The model under review builds one solid part; all positions refer to its coordinate system, in mm. Round coordinates to 2 decimals unless told otherwise and drop trailing zeros.
```python
from build123d import *

# Parameters (mm, degrees)
SKETCH1_W           = 368.3
SKETCH1_H           = 292.1
SKETCH1_R           = 99.3775
SKETCH1_R_2         = 2.54
BOSS_EXTRUDE1_DEPTH = 6.35
SKETCH2_R           = 14.2875
SKETCH2_R_2         = 2.38125
CUT_EXTRUDE1_DEPTH  = 7.35
FILLET1_R           = 12.7


with BuildPart() as part:
    # Sketch1 → Boss-Extrude1 (new body)
    with BuildSketch(Plane.XY):
        with Locations((184.15, 146.05)):
            Rectangle(SKETCH1_W, SKETCH1_H)
        with Locations((179.07, 138.43)):
            Circle(SKETCH1_R, mode=Mode.SUBTRACT)
        with Locations((12.7, 279.4)):
            Circle(SKETCH1_R_2, mode=Mode.SUBTRACT)
        with Locations((25.4, 279.4)):
            Circle(SKETCH1_R_2, mode=Mode.SUBTRACT)
        with Locations((38.1, 279.4)):
            Circle(SKETCH1_R_2, mode=Mode.SUBTRACT)
        with Locations((50.8, 279.4)):
            Circle(SKETCH1_R_2, mode=Mode.SUBTRACT)
        with Locations((63.5, 279.4)):
            Circle(SKETCH1_R_2, mode=Mode.SUBTRACT)
        with Locations((76.2, 279.4)):
            Circle(SKETCH1_R_2, mode=Mode.SUBTRACT)
        with Locations((88.9, 279.4)):
            Circle(SKETCH1_R_2, mode=Mode.SUBTRACT)
        with Locations((101.6, 279.4)):
            Circle(SKETCH1_R_2, mode=Mode.SUBTRACT)
        with Locations((114.3, 279.4)):
            Circle(SKETCH1_R_2, mode=Mode.SUBTRACT)
        with Locations((127, 279.4)):
            Circle(SKETCH1_R_2, mode=Mode.SUBTRACT)
        with Locations((139.7, 279.4)):
            Circle(SKETCH1_R_2, mode=Mode.SUBTRACT)
        with Locations((152.4, 279.4)):
            Circle(SKETCH1_R_2, mode=Mode.SUBTRACT)
        with Locations((165.1, 279.4)):
            Circle(SKETCH1_R_2, mode=Mode.SUBTRACT)
        with Locations((177.8, 279.4)):
            Circle(SKETCH1_R_2, mode=Mode.SUBTRACT)
        with Locations((190.5, 279.4)):
            Circle(SKETCH1_R_2, mode=Mode.SUBTRACT)
        with Locations((203.2, 279.4)):
            Circle(SKETCH1_R_2, mode=Mode.SUBTRACT)
        with Locations((215.9, 279.4)):
            Circle(SKETCH1_R_2, mode=Mode.SUBTRACT)
        with Locations((228.6, 279.4)):
            Circle(SKETCH1_R_2, mode=Mode.SUBTRACT)
        with Locations((12.7, 266.7)):
            Circle(SKETCH1_R_2, mode=Mode.SUBTRACT)
        with Locations((12.7, 254)):
            Circle(SKETCH1_R_2, mode=Mode.SUBTRACT)
        with Locations((12.7, 241.3)):
            Circle(SKETCH1_R_2, mode=Mode.SUBTRACT)
        with Locations((12.7, 228.6)):
            Circle(SKETCH1_R_2, mode=Mode.SUBTRACT)
        with Locations((12.7, 215.9)):
            Circle(SKETCH1_R_2, mode=Mode.SUBTRACT)
        with Locations((12.7, 203.2)):
            Circle(SKETCH1_R_2, mode=Mode.SUBTRACT)
        with Locations((12.7, 190.5)):
            Circle(SKETCH1_R_2, mode=Mode.SUBTRACT)
        with Locations((12.7, 177.8)):
            Circle(SKETCH1_R_2, mode=Mode.SUBTRACT)
        with Locations((12.7, 165.1)):
            Circle(SKETCH1_R_2, mode=Mode.SUBTRACT)
        with Locations((12.7, 152.4)):
            Circle(SKETCH1_R_2, mode=Mode.SUBTRACT)
        with Locations((12.7, 139.7)):
            Circle(SKETCH1_R_2, mode=Mode.SUBTRACT)
        with Locations((12.7, 127)):
            Circle(SKETCH1_R_2, mode=Mode.SUBTRACT)
        with Locations((12.7, 114.3)):
            Circle(SKETCH1_R_2, mode=Mode.SUBTRACT)
        with Locations((12.7, 101.6)):
            Circle(SKETCH1_R_2, mode=Mode.SUBTRACT)
        with Locations((12.7, 88.9)):
            Circle(SKETCH1_R_2, mode=Mode.SUBTRACT)
        with Locations((12.7, 76.2)):
            Circle(SKETCH1_R_2, mode=Mode.SUBTRACT)
        with Locations((12.7, 63.5)):
            Circle(SKETCH1_R_2, mode=Mode.SUBTRACT)
        with Locations((12.7, 50.8)):
            Circle(SKETCH1_R_2, mode=Mode.SUBTRACT)
        with Locations((12.7, 38.1)):
            Circle(SKETCH1_R_2, mode=Mode.SUBTRACT)
        with Locations((12.7, 25.4)):
            Circle(SKETCH1_R_2, mode=Mode.SUBTRACT)
        with Locations((12.7, 12.7)):
            Circle(SKETCH1_R_2, mode=Mode.SUBTRACT)
        with Locations((25.4, 12.7)):
            Circle(SKETCH1_R_2, mode=Mode.SUBTRACT)
        with Locations((38.1, 12.7)):
            Circle(SKETCH1_R_2, mode=Mode.SUBTRACT)
        with Locations((50.8, 12.7)):
            Circle(SKETCH1_R_2, mode=Mode.SUBTRACT)
        with Locations((63.5, 12.7)):
            Circle(SKETCH1_R_2, mode=Mode.SUBTRACT)
        with Locations((76.2, 12.7)):
            Circle(SKETCH1_R_2, mode=Mode.SUBTRACT)
        with Locations((88.9, 12.7)):
            Circle(SKETCH1_R_2, mode=Mode.SUBTRACT)
        with Locations((101.6, 12.7)):
            Circle(SKETCH1_R_2, mode=Mode.SUBTRACT)
        with Locations((114.3, 12.7)):
            Circle(SKETCH1_R_2, mode=Mode.SUBTRACT)
        with Locations((127, 12.7)):
            Circle(SKETCH1_R_2, mode=Mode.SUBTRACT)
        with Locations((139.7, 12.7)):
            Circle(SKETCH1_R_2, mode=Mode.SUBTRACT)
        with Locations((152.4, 12.7)):
            Circle(SKETCH1_R_2, mode=Mode.SUBTRACT)
        with Locations((165.1, 12.7)):
            Circle(SKETCH1_R_2, mode=Mode.SUBTRACT)
        with Locations((177.8, 12.7)):
            Circle(SKETCH1_R_2, mode=Mode.SUBTRACT)
        with Locations((190.5, 12.7)):
            Circle(SKETCH1_R_2, mode=Mode.SUBTRACT)
        with Locations((203.2, 12.7)):
            Circle(SKETCH1_R_2, mode=Mode.SUBTRACT)
        with Locations((215.9, 12.7)):
            Circle(SKETCH1_R_2, mode=Mode.SUBTRACT)
        with Locations((228.6, 12.7)):
            Circle(SKETCH1_R_2, mode=Mode.SUBTRACT)
        with Locations((241.3, 12.7)):
            Circle(SKETCH1_R_2, mode=Mode.SUBTRACT)
        with Locations((254, 12.7)):
            Circle(SKETCH1_R_2, mode=Mode.SUBTRACT)
        with Locations((266.7, 12.7)):
            Circle(SKETCH1_R_2, mode=Mode.SUBTRACT)
        with Locations((279.4, 12.7)):
            Circle(SKETCH1_R_2, mode=Mode.SUBTRACT)
    extrude(amount=BOSS_EXTRUDE1_DEPTH)

    # Sketch2 → Cut-Extrude1 (cut, through all)
    with BuildSketch(Plane.XY.offset(6.35)):
        with Locations((62.079722251, 62.079722251)):
            Circle(SKETCH2_R)
        with Locations((269.10870269, 245.243491741)):
            Circle(SKETCH2_R)
        with Locations((62.079722251, 87.479722251)):
            Circle(SKETCH2_R_2)
        with Locations((80.040234493, 80.040234493)):
            Circle(SKETCH2_R_2)
        with Locations((87.479722251, 62.079722251)):
            Circle(SKETCH2_R_2)
        with Locations((80.040234493, 44.119210009)):
            Circle(SKETCH2_R_2)
        with Locations((62.079722251, 36.679722251)):
            Circle(SKETCH2_R_2)
        with Locations((44.119210009, 44.119210009)):
            Circle(SKETCH2_R_2)
        with Locations((36.679722251, 62.079722251)):
            Circle(SKETCH2_R_2)
        with Locations((44.119210009, 80.040234493)):
            Circle(SKETCH2_R_2)
        with Locations((269.10870269, 270.643491741)):
            Circle(SKETCH2_R_2)
        with Locations((287.069214932, 263.204003983)):
            Circle(SKETCH2_R_2)
        with Locations((294.50870269, 245.243491741)):
            Circle(SKETCH2_R_2)
        with Locations((287.069214932, 227.282979499)):
            Circle(SKETCH2_R_2)
        with Locations((269.10870269, 219.843491741)):
            Circle(SKETCH2_R_2)
        with Locations((251.148190448, 227.282979499)):
            Circle(SKETCH2_R_2)
        with Locations((243.70870269, 245.243491741)):
            Circle(SKETCH2_R_2)
        with Locations((251.148190448, 263.204003983)):
            Circle(SKETCH2_R_2)
    extrude(amount=-CUT_EXTRUDE1_DEPTH, mode=Mode.SUBTRACT)

    # Fillet1
    fillet1_edges = [part.edges().sort_by_distance(p)[0] for p in [
        (0, 292.1, 3.175),
        (368.3, 292.1, 3.175),
        (368.3, 0, 3.175),
        (0, 0, 3.175),
    ]]
    fillet(fillet1_edges, radius=FILLET1_R)


solid = part.part
```
(1) Draft analysis for pull direction X (two halves, no side actions). For faces 1 (the cylindrical face through (364.48, 288.48, 3.22)), 2 (the flat face through (182, 245, 6.35)), 3 (the cylindrical face through (257.77, 236.55, 3.22)), state which applies: pulls with the +X half, pulls with the -X half, needs draft (parallel to the pull), parting line crosses it, or undercut.
Data:
face 1: pulls with the +X half
face 2: needs draft
face 3: undercut
(2) Consider section A-A (z = 5). State how many separate pieces and enclosed holes the cut face has, and give its area (3 significant figures).
Data:
separate pieces: 1
enclosed holes: 79
area: 73,600 mm2
(3) Insertion check: pin 1 (7.5 mm diameter, centred on x = 80.04, y = 44.12, fed in from +Z). The pin has a flat end and moves straight along its axis. Give the tip position at first contact, or say it passes through.
Data:
pin 1: stops at z = 6.35
(4) To check wall thickness, follow probe 1 along Y at (x, z) = (177.5, 6.25); probe 2 along X at (y, z) = (64.5, 5.5); probe 3 along Y at (x, z) = (91, 4). State the ranges of each line that lie inside material, in increasing order.
Data:
probe 1: y = 0 to 10.18, 15.22 to 39.06, 237.8 to 276.88, 281.92 to 292.1
probe 2: x = 0 to 10.37, 15.03 to 48, 76.16 to 112.66, 245.48 to 368.3
probe 3: y = 0 to 11.27, 14.13 to 92.39, 184.47 to 277.97, 280.83 to 292.1
